Design review of the part built by this model. Coordinates are the model's own, in mm. A direction names the side the tool comes from. Give positions to 0.01 mm unless a question says otherwise; leave off trailing zeros. Order: outer loops, then holes, each group sorted by start corner. A loop starts at its lowest first (then second) coordinate and runs counter-clockwise, first axis right, second up. Notation, with made-up numbers: M -9,76.5 L 17,76.5 A29 ccw 17,110.5 Z; hole C 87.25,-30 d7. An arc over 180 degrees is marked long. Answer as a JSON object with one key per item and string values.
Autodesk Inventor part; units mm, degrees
ref_plane "YZ Plane" through (0, 0, 0) normal (1, 0, 0) x (0, 1, 0)
ref_plane "XZ Plane" through (0, 0, 0) normal (0, 1, 0) x (-1, 0, 0)
ref_plane "XY Plane" through (0, 0, 0) normal (0, 0, 1) x (1, 0, 0)
sketch "草图1" plane through (0, 0, 0) normal (0, 0, 1) x (1, 0, 0)
  line L0 (-35, 65) -> (35, 65)
  line L1 (35, 65) -> (35, -65)
  line L2 (35, -65) -> (-35, -65)
  line L3 (-35, -65) -> (-35, 65)
  line L4 (-35, 65) -> (35, -65) construction
  line L5 (35, 65) -> (-35, -65) construction
  point P0 (0, 0)
  dimension "d0" = 70
  dimension "d1" = 130
extrude "拉伸1" add sketch "草图1" along normal blind 1000
sketch "草图2" plane through (-35, -65, 0) normal (-1, 0, 0) x (0, 0, 1)
  line L0 (0, 65) -> (300, 0)
  line L1 (0, 0) -> (1000, 0)
  line L2 (0, 130) -> (1000, 130)
  line L3 (300, 130) -> (0, 65)
  line L4 (300, 0) -> (300, 130)
  line L5 (0, 0) -> (0, 130)
  dimension "d4" = 300
extrude "拉伸2" cut sketch "草图2" against normal through all contours L5 L2 L3 | L0 L1 L5
fillet "圆角1" radius 30 3 edges at (0, 0, 0) (0, 65, 300) (0, -65, 300)
sketch "草图3" plane through (-35, -65, 1000) normal (-1, 0, 0) x (0, 0, 1)
  arc A0 (-864.6783, 94.3197) -> (-864.6783, 35.6803) centre (-858.3257, 65) ccw
  circle A1 centre (-858.3257, 65) radius 15
  circle A2 centre (-758.3257, 65) radius 15
  point P0 (-1000, 65)
  dimension "d8" = 30
  dimension "d11" = 30
  dimension "d12" = 100
extrude "拉伸3" cut sketch "草图3" against normal through all
sketch "草图4" plane through (0, 0, 1000) normal (0, 0, 1) x (1, 0, 0)
  line L0 (-53.3891, 25) -> (64.6192, 25)
  line L1 (0, 81.4777) -> (0, 16.0102)
  line L2 (-20, 45) -> (20, 45)
  line L3 (20, 45) -> (20, 5)
  line L4 (20, 5) -> (-20, 5)
  line L5 (-20, 5) -> (-20, 45)
  line L6 (-20, 45) -> (20, 5) construction
  line L7 (20, 45) -> (-20, 5) construction
  line L8 (35, 65) -> (-35, 65)
  point P0 (0, 0)
  point P1 (0, 25)
  dimension "d13" = 40
  dimension "d14" = 40
  dimension "d15" = 40
extrude "拉伸4" cut sketch "草图4" against normal blind 700
sketch "草图5" plane through (-20, 5, 1000) normal (1, 0, 0) x (0, 0, -1)
  line L0 (-16.4327, 20) -> (719.4245, 20)
  line L1 (696.7873, 60) -> (0, 60)
  circle A0 centre (650, 20) radius 15
  line L2 (0, -70) -> (0, 60)
  point P0 (1000, -5)
  dimension "d18" = 40
  dimension "d19" = 30
  dimension "d20" = 650
extrude "拉伸5" cut sketch "草图5" along normal mid plane 700
sketch "草图6" plane through (0, 0, 0) normal (1, 0, 0) x (0, 1, 0)
  circle A0 centre (95, 800) radius 15
  line L0 (65, 303.2127) -> (65, 1000)
  line L1 (-65, 1000) -> (65, 1000)
  line L2 (95.8043, 829.9892) -> (131.374, 829.9892) construction
  line L3 (109.6775, 773.8357) -> (183.0515, 773.8357) construction
  line L4 (65, 847.7741) -> (65, 745.182)
  circle A1 centre (95, 800) radius 30
  line L5 (110.3646, 825.7668) -> (65, 851.9581)
  line L6 (110.3646, 825.7668) -> (162.747, 825.7668) construction
  line L7 (65, 851.9581) -> (65, 745.182)
  line L8 (65, 303.2127) -> (65, 1000)
  line L9 (111.8573, 775.184) -> (65, 748.131)
  line L10 (111.8573, 775.184) -> (168.7185, 775.184) construction
  point P0 (0, 0)
  dimension "d23" = 30
  dimension "d25" = 30
  dimension "d26" = 200
  dimension "d29" = 60
  dimension "d30" = 150
  dimension "d31" = 150
extrude "拉伸6" add sketch "草图6" along normal mid plane 70
sketch "草图7" plane through (-35, 65, 1000) normal (0, 1, 0) x (1, 0, 0)
  line L0 (70, 148.0419) -> (0, 148.0419)
  line L1 (35, 148.0419) -> (35, 251.869)
  line L2 (0, 251.869) -> (70, 251.869)
  line L3 (0, 185) -> (0, 215)
  line L4 (0, 200) -> (70.1178, 200)
  line L5 (17.5589, 104.0655) -> (52.5589, 104.0655)
  line L6 (52.5589, 104.0655) -> (52.5589, 295.9345)
  line L7 (52.5589, 295.9345) -> (17.5589, 295.9345)
  line L8 (17.5589, 295.9345) -> (17.5589, 104.0655)
  line L9 (17.5589, 104.0655) -> (52.5589, 295.9345) construction
  line L10 (52.5589, 104.0655) -> (17.5589, 295.9345) construction
  point P0 (35, 1000)
  point P1 (35.0589, 200)
  dimension "d35" = 35
extrude "拉伸7" cut sketch "草图7" along normal blind 70
properties part number "DipperSon" material "钢，高强度，低合金"
(1) Insertion check: pin 1 (18 mm diameter, centred on y = 0, z = 241.67, fed in from +X); pin 2 (4 mm diameter, centred on x = -21, z = 342, fed in from +Y); pin 3 (12 mm diameter, centred on x = -8.5, y = 17.5, fed in from +Z); pin 4 (5 mm diameter, centred on x = 18.5, y = 99.5, fed in from -Z). Each pin has a flat end and moves straight along its axis. Give the tip position at first contact, or say it passes through.
Checked values:
{"pin 1": "passes through", "pin 2": "stops at y = 65", "pin 3": "stops at z = 300", "pin 4": "stops at z = 766.61"}
(2) Tool access review of faces 1 (the flat face through (-20, 25, 655)), 2 (the flat face through (26.16, 88, 838.68)), 3 (the flat face through (17.559, 81, 789)): name each direction out of +Z, -Z, +X, -X, +Y, -Y from which nothing blocks a thin tool from reaching the whole face with its end or side.
Checked values:
{"face 1": "+Z", "face 2": "+Z, +X, -X, +Y", "face 3": "+Z, -Z, +Y"}
(3) We need section A-A (z = 800). Write out the cut boundary in (x, y).
Checked values:
{"outline": "M -35,-65 L 35,-65 L 35,80 L 17.56,80 L 17.56,65 L -17.44,65 L -17.44,80 L -35,80 Z; M -35,110 L -17.44,110 L -17.44,125 L -35,125 Z; M 17.56,110 L 35,110 L 35,125 L 17.56,125 Z; hole M -20,5 L 20,5 L 20,45 L -20,45 Z"}
(4) We need section C-C (z = 350). Write out the cut boundary in (x, y).
Checked values:
{"outline": "M -35,-65 L 35,-65 L 35,10 L 20,10 L 20,5 L -20,5 L -20,10 L -35,10 Z; M -35,40 L -20,40 L -20,45 L 20,45 L 20,40 L 35,40 L 35,65 L -35,65 Z"}
(5) We need section B-B (x = 9.5). Write out the cut boundary in (y, z).
Checked values:
{"outline": "M -65,303.21 A30 ccw -64.32,296.86 L -29.32,135.32 A30 ccw 29.32,135.32 L 64.32,296.86 A30 ccw 65,303.21 L 65,1000 L 45,1000 L 45,300 L 5,300 L 5,1000 L -65,1000 Z; hole C 0,141.67 d30; hole C 0,241.67 d30"}
(6) To check wall thickness, follow L1, parallel to X at y = 23.5, z = 559; L2, parallel to Z at x = -7, y = -9.5; L3, parallel to X at y = 96, z = 825. State the ranges of each line that lie inside material, in increasing order. Write a range as from..to.
Checked values:
{"L1": "x = -35..-20, 20..35", "L2": "z = 113.22..130.07, 153.28..230.07, 253.28..1000", "L3": "x = -35..-17.44, 17.56..35"}
(7) We need section D-D (z = 680.5). Write out the cut boundary in (x, y), plus the area to 3 significant figures.
Checked values:
{"outline": "M -35,-65 L 35,-65 L 35,65 L -35,65 Z; hole M -20,5 L 20,5 L 20,45 L -20,45 Z", "area": "7,500 mm^2"}
(8) Draft analysis for pull direction Z (two halves, no side actions). For faces 4 (the cylindrical face through (-26.343, 124.988, 799.145)), 5 (the flat face through (-26.34, 88, 838.68)), 6 (the cylindrical face through (-0.49, 0.66, 226.69)), 7 (the cylindrical face through (-0.49, 4.51, 155.98)), state which applies: +Z half, -Z half, draft (parallel to the pull), parting line (faces both ways), or undercut.
Checked values:
{"face 4": "parting line", "face 5": "+Z half", "face 6": "undercut", "face 7": "undercut"}
